Source: CAD feature listing. Evaluate the final solid. Frame: model axes, mm. A direction names the side the tool comes from. Give positions to 0.01 mm unless a question says otherwise; leave off trailing zeros. Write each loop counter-clockwise with the first axis right and the second up, starting at its lowest first coordinate (ties: lowest second). Pieces come first, ordered by that corner, then holes. Notation, with made-up numbers: M -35.5,-40 L -6.5,-40 A27 ccw -6.5,-7 Z; hole C 4,89.5 d2. An arc over 180 degrees is marked long. Return JSON: item names as keys, results as strings.
```python
from build123d import *

# Parameters (mm, degrees)
BOSS_EXTRUDE1_DEPTH = 1.96
SKETCH2_R           = 18.76
BOSS_EXTRUDE2_DEPTH = 1.96
SKETCH3_R           = 28.461143805
BOSS_EXTRUDE3_DEPTH = 1.96
CUT_EXTRUDE1_REACH  = 42.441
SKETCH4_R           = 1.25
CUT_EXTRUDE2_REACH  = 42.441
SKETCH5_R           = 4.205
SKETCH5_R_2         = 1.75
SKETCH6_R           = 6.75
CUT_EXTRUDE3_DEPTH  = 1.42


with BuildPart() as part:
    # Sketch1 → Boss-Extrude1 (new body)
    with BuildSketch(Plane(origin=(0, 0, 0), x_dir=(1, 0, 0), z_dir=(0, 1, 0))):
        with BuildLine():
            Line((-2.18, 22.175), (-2.18, -22.175))
            ThreePointArc((-2.18, -22.175), (0, -24.355), (2.18, -22.175))
            Line((2.18, -22.175), (2.18, 22.175))
            ThreePointArc((2.18, 22.175), (0, 24.355), (-2.18, 22.175))
        make_face()
    extrude(amount=BOSS_EXTRUDE1_DEPTH)

    # Sketch2 → Boss-Extrude2 (add)
    with BuildSketch(Plane.XZ):
        Circle(SKETCH2_R)
    extrude(amount=-BOSS_EXTRUDE2_DEPTH)

    # Sketch3 → Boss-Extrude3 (add)
    with BuildSketch(Plane.XZ):
        with Locations(Location((0, 0, 0), (0, 0, 270))):
            Circle(SKETCH3_R)
    extrude(amount=BOSS_EXTRUDE3_DEPTH)

    # Sketch4 → Cut-Extrude1 (cut, up to next)
    with BuildSketch(Plane(origin=(0, 1.96, 0), x_dir=(1, 0, 0), z_dir=(0, 1, 0)), mode=Mode.PRIVATE) as cut_extrude1_sk1:
        with Locations(Location((0, 22.175, 0), (0, 0, 270))):
            Circle(SKETCH4_R)
    cut_extrude1_tool1 = extrude(cut_extrude1_sk1.sketch, amount=-CUT_EXTRUDE1_REACH, mode=Mode.PRIVATE) & part.part
    # Sketch4 → Cut-Extrude1 (cut, up to next)
    with BuildSketch(Plane(origin=(0, 1.96, 0), x_dir=(1, 0, 0), z_dir=(0, 1, 0)), mode=Mode.PRIVATE) as cut_extrude1_sk2:
        with Locations(Location((0, -22.175, 0), (0, 0, 270))):
            Circle(SKETCH4_R)
    cut_extrude1_tool2 = extrude(cut_extrude1_sk2.sketch, amount=-CUT_EXTRUDE1_REACH, mode=Mode.PRIVATE) & part.part
    add(cut_extrude1_tool1.solids().sort_by_distance((0, 1.96, -22.175))[0], mode=Mode.SUBTRACT)
    add(cut_extrude1_tool2.solids().sort_by_distance((0, 1.96, 22.175))[0], mode=Mode.SUBTRACT)

    # Sketch5 → Cut-Extrude2 (cut, up to next)
    with BuildSketch(Plane(origin=(0, 1.96, 0), x_dir=(1, 0, 0), z_dir=(0, 1, 0)), mode=Mode.PRIVATE) as cut_extrude2_sk1:
        with Locations(Location((0, 0, 0), (0, 0, 270))):
            Circle(SKETCH5_R)
    cut_extrude2_tool1 = extrude(cut_extrude2_sk1.sketch, amount=-CUT_EXTRUDE2_REACH, mode=Mode.PRIVATE) & part.part
    # Sketch5 → Cut-Extrude2 (cut, up to next)
    with BuildSketch(Plane(origin=(0, 1.96, 0), x_dir=(1, 0, 0), z_dir=(0, 1, 0)), mode=Mode.PRIVATE) as cut_extrude2_sk2:
        with Locations(Location((0, 9.975, 0), (0, 0, 270))):
            Circle(SKETCH5_R_2)
    cut_extrude2_tool2 = extrude(cut_extrude2_sk2.sketch, amount=-CUT_EXTRUDE2_REACH, mode=Mode.PRIVATE) & part.part
    add(cut_extrude2_tool1.solids().sort_by_distance((0, 1.96, 0))[0], mode=Mode.SUBTRACT)
    add(cut_extrude2_tool2.solids().sort_by_distance((0, 1.96, -9.975))[0], mode=Mode.SUBTRACT)

    # Sketch6 → Cut-Extrude3 (cut)
    with BuildSketch(Plane.XZ.offset(1.96)):
        with Locations(Location((0, 0, 0), (0, 0, 270))):
            Circle(SKETCH6_R)
    extrude(amount=-CUT_EXTRUDE3_DEPTH, mode=Mode.SUBTRACT)


solid = part.part
```
1) Cut plane B-B, the plane z = 0. Return the cut outline in (x, y) (3 decimals), then the cut area to 3 significant figures.
Numbers:
{"outline": "M -28.461,-1.96 L -6.75,-1.96 L -6.75,-0.54 L -4.205,-0.54 L -4.205,1.96 L -18.76,1.96 L -18.76,0 L -28.461,0 Z; M 4.205,-0.54 L 6.75,-0.54 L 6.75,-1.96 L 28.461,-1.96 L 28.461,0 L 18.76,0 L 18.76,1.96 L 4.205,1.96 Z", "area": "145 mm²"}
2) Draft query along Z for faces 6 (the face through (0.055, 0.027, 20.926)), 7 (the face through (1.183, 0.027, -11.265)), 8 (the face through (-4.4, 1.96, 0.3)), 9 (the face through (-27.784, -0.966, 6.17)). Return one class per face: released by +Z, released by -Z, zero draft, split by the parting line, or undercut.
Numbers:
{"face 6": "undercut", "face 7": "undercut", "face 8": "zero draft", "face 9": "split by the parting line"}
3) Cut plane A-A, the plane x = 0. Return the cut outline in (y, z) (3 decimals), then the cut area to 3 significant figures.
Numbers:
{"outline": "M -1.96,-28.461 L 0,-28.461 L 0,-24.355 L 1.96,-24.355 L 1.96,-23.425 L -1.96,-23.425 Z; M -1.96,-20.925 L 1.96,-20.925 L 1.96,-11.725 L -1.96,-11.725 Z; M -1.96,-8.225 L 1.96,-8.225 L 1.96,-4.205 L -0.54,-4.205 L -0.54,-6.75 L -1.96,-6.75 Z; M -1.96,6.75 L -0.54,6.75 L -0.54,4.205 L 1.96,4.205 L 1.96,20.925 L -1.96,20.925 Z; M -1.96,23.425 L 1.96,23.425 L 1.96,24.355 L 0,24.355 L 0,28.461 L -1.96,28.461 Z", "area": "134 mm²"}
4) Cut plane D-D, the plane z = -10. Return the cut outline in (x, y).
Numbers:
{"outline": "M -26.65,-1.96 L -1.75,-1.96 L -1.75,1.96 L -15.87,1.96 L -15.87,0 L -26.65,0 Z; M 1.75,-1.96 L 26.65,-1.96 L 26.65,0 L 15.87,0 L 15.87,1.96 L 1.75,1.96 Z"}
5) Cut plane C-C, the plane y = 0.8. Return the cut outline in (x, z) (3 decimals), then the cut area to 3 significant figures.
Numbers:
{"outline": "M -2.18,-22.175 A2.18 ccw 2.18,-22.175 L 2.18,-18.633 A18.76 ccw 2.18,18.633 L 2.18,22.175 A2.18 ccw -2.18,22.175 L -2.18,18.633 A18.76 ccw -2.18,-18.633 Z; hole C 0,0 d8.41; hole C 0,-9.975 d3.5; hole C 0,-22.175 d2.5; hole C 0,22.175 d2.5", "area": "1,080 mm²"}
6) Set-up query: faces 1 (the face through (2.18, 1, -20)), 2 (the face through (-2.18, 1, -20)), 3 (the face through (-2.18, 1, 20)), 4 (the face through (18.756, 0.966, -0.382)), 5 (the face through (-6.59, -1.26, 1.46)). Return all of +Z, -Z, +X, -X, +Y, -Y with unobstructed straight access to the full face (end or side cutting, diameter ignored); none if empty.
Numbers:
{"face 1": "-Z, +X, +Y", "face 2": "-Z, -X, +Y", "face 3": "+Z, -X, +Y", "face 4": "+X, +Y", "face 5": "-Y"}
7) Line query: line 1 (X direction, y = 0.75, z = 0) (3 decimals); line 2 (X direction, y = -0.9, z = 0); line 3 (Z direction, x = 0.5, y = -0.1). Output: solid intervals per line, ascending. Write a range as [from, to].
Numbers:
{"line 1": "x = [-18.76, -4.205], [4.205, 18.76]", "line 2": "x = [-28.46, -6.75], [6.75, 28.46]", "line 3": "z = [-28.46, -23.32], [-21.03, -11.65], [-8.3, -4.18], [4.18, 21.03], [23.32, 28.46]"}
8) Contact query for flat-ended pins moving along their axis: pin 1 Ø9.5 at (x, z) = (0, 0) entering from -Y; pin 2 Ø1.6 at (y, z) = (0.5, -21) entering from -X; pin 3 Ø1.6 at (y, z) = (1, 20.5) entering from -X. Output: stop coordinate, or through.
Numbers:
{"pin 1": "stops at y = -0.54", "pin 2": "stops at x = -19.87", "pin 3": "stops at x = -2.18"}
